For this review, take the finished solid that the model builds, in its own axes (mm). Face numbers are marked on the shaded views. A direction names the side the tool comes from. Coordinates: 2 decimals unless noted, no trailing zeros. Loops run counter-clockwise (first coordinate to the right, second up) from the corner with the lowest first, then second, coordinate; pieces in that order, holes last. Notation, with made-up numbers: (-16, -22.5) -> (-2, -22.5) arc R32 ccw to (-2, 5.5) -> close; hole circle Ø8 at (51, 84). An arc over 180 degrees is marked (long way). Answer in a Markdown table with one row per item.
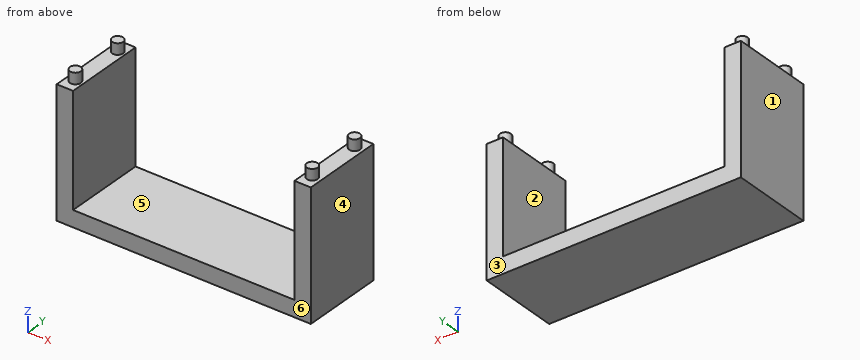
from build123d import *

# Parameters (mm, degrees)
BOSS_EXTRUDE2_DEPTH = 15
SKETCH4_R           = 1
BOSS_EXTRUDE3_DEPTH = 2


with BuildPart() as part:
    # Sketch2 → Boss-Extrude2 (new body)
    with BuildSketch(Plane(origin=(0, 0, 0), x_dir=(1, 0, 0), z_dir=(0, 1, 0))):
        Polygon((0, 0), (0, 23.5), (46.6, 23.5), (46.6, 0), (43.6, 0), (43.6, 20.5), (3, 20.5), (3, 0), align=None)
    extrude(amount=BOSS_EXTRUDE2_DEPTH)

    # Sketch4 → Boss-Extrude3 (add)
    with BuildSketch(Plane.XY):
        with Locations(Location((1.583, 2.42, 0), (0, 0, 180))):
            Circle(SKETCH4_R)
        with Locations(Location((1.583, 12.58, 0), (0, 0, 180))):
            Circle(SKETCH4_R)
        with Locations(Location((45.017, 12.58, 0), (0, 0, 180))):
            Circle(SKETCH4_R)
        with Locations(Location((45.017, 2.42, 0), (0, 0, 180))):
            Circle(SKETCH4_R)
    extrude(amount=BOSS_EXTRUDE3_DEPTH)


solid = part.part
Item 1: The part is to be moulded in two halves that separate along X. For the marked faces 1, 2, 3 and 4, say which applies: +X half, -X half, draft (parallel to the pull), parting line (faces both ways), or undercut.
Worked answers:
| item | result |
|---|---|
| face 1 | -X half |
| face 2 | undercut |
| face 3 | draft |
| face 4 | +X half |
Item 2: Insertion check: pin 1 (2.5 mm diameter, centred on x = 1.5, y = 5, fed in from +Z); pin 2 (4.5 mm diameter, centred on x = 31, y = 8.5, fed in from +Z). Each pin has a flat end and moves straight along its axis. Give the tip position at first contact, or say it passes through.
Worked answers:
| item | result |
|---|---|
| pin 1 | z = 0 |
| pin 2 | z = -20.5 |
Item 3: For L1, parallel to X at y = 6.5, z = -19.75; L2, parallel to Z at x = 19, y = 4.75; L3, parallel to Z at x = 45, y = 10.5, list the stretches that pass through material, from the lowest coordinate up.
Worked answers:
| item | result |
|---|---|
| L1 | 0 to 3, 43.6 to 46.6 |
| L2 | -23.5 to -20.5 |
| L3 | -23.5 to 0 |
Item 4: Take a section at B-B, the plane y = 2.42. State the section outline as (x, z) points.
Worked answers:
| item | result |
|---|---|
| outline | (0, -23.5) -> (46.6, -23.5) -> (46.6, 0) -> (46.02, 0) -> (46.02, 2) -> (44.02, 2) -> (44.02, 0) -> (43.6, 0) -> (43.6, -20.5) -> (3, -20.5) -> (3, 0) -> (2.58, 0) -> (2.58, 2) -> (0.58, 2) -> (0.58, 0) -> (0, 0) -> close |
Item 5: Take a section at D-D, the plane y = 6.75. State the section outline as (x, z) points.
Worked answers:
| item | result |
|---|---|
| outline | (0, -23.5) -> (46.6, -23.5) -> (46.6, 0) -> (43.6, 0) -> (43.6, -20.5) -> (3, -20.5) -> (3, 0) -> (0, 0) -> close |
Item 6: For the marked faces 5 and 6, list the 3-axis set-ups (+Z, -Z, +X, -X, +Y, -Y) from which the entire face can be reached by the end or side of a thin tool; tool diameter is ignored.
Worked answers:
| item | result |
|---|---|
| face 5 | +Z, +Y, -Y |
| face 6 | +Z, -Z, +X, -X, -Y |
Item 7: Take a section at A-A, the plane z = -0.5. State the section outline as (x, y) points.
Worked answers:
| item | result |
|---|---|
| outline | (0, 0) -> (3, 0) -> (3, 15) -> (0, 15) -> close; (43.6, 0) -> (46.6, 0) -> (46.6, 15) -> (43.6, 15) -> close |
Item 8: Take a section at C-C, the plane x = 24.5. State the section outline as (y, z) points.
Worked answers:
| item | result |
|---|---|
| outline | (0, -23.5) -> (15, -23.5) -> (15, -20.5) -> (0, -20.5) -> close |
